Can you work these out from the model? Positions are in its coordinate system, mm. Face numbers are marked on the shaded views. Give positions to 0.01 mm unless a question says otherwise; leave off trailing zeros. Loops run counter-clockwise (first coordinate to the right, second up) from the corner with the lowest first, then second, coordinate; pieces in that order, holes last. Notation, with made-up numbers: (86, -5.75) - (128, -5.75) arc R19 ccw to (128, 30.25) - close; hole circle Ø10 at (-20.75, 38). An arc over 180 degrees is marked (long way). Answer as a JSON object with one key per item and string values.
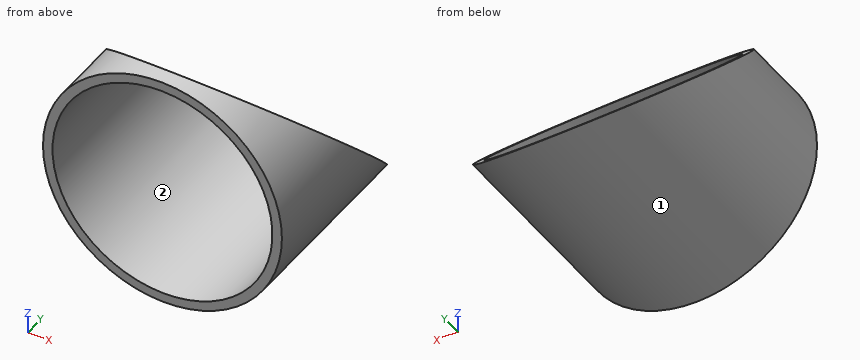
```python
from build123d import *

# Parameters (mm, degrees)
SKETCH2_R               = 20
BOSS_EXTRUDE1_DEPTH     = 0.707106781
SKETCH3_R               = 7.4
SKETCH3_R_2             = 5.9
BOSS_EXTRUDE2_DEPTH     = 1
CUT_EXTRUDE1_DEPTH      = 48.148112734
CUT_EXTRUDE1_DEPTH_BACK = 48.148112734
SKETCH4_W               = 305.220008054
SKETCH4_H               = 126.870977102
SKETCH4_R               = 6.4
BOSS_EXTRUDE3_REACH     = 25.052
SKETCH5_R               = 6.28
SKETCH5_R_2             = 5.78
SKETCH7_R               = 18.282703858
CUT_EXTRUDE3_DEPTH      = 0.707106781
SKETCH8_R               = 12.772794789
CUT_EXTRUDE4_DEPTH      = 2.52


with BuildPart() as part:
    # Sketch2 → Boss-Extrude1 (new body)
    with BuildSketch(Plane(origin=(0, 0, 0), x_dir=(1, 0, 0), z_dir=(0, 0.7071067811865464, 0.7071067811865488))):
        with Locations(Location((0, 20, 0), (0, 0, 270))):
            Circle(SKETCH2_R)
    extrude(amount=-BOSS_EXTRUDE1_DEPTH)

    # Sketch4 → Cut-Extrude1 (cut, two sides: drawn at the far end of the back side and taken through both)
    with BuildSketch(Plane.XZ.offset(3.25).offset(-CUT_EXTRUDE1_DEPTH_BACK)):
        with Locations((6.754756468, -15.87939177)):
            Rectangle(SKETCH4_W, SKETCH4_H)
        with Locations(Location((0, -7.4, 0), (0, 0, 90))):
            Circle(SKETCH4_R, mode=Mode.SUBTRACT)
    extrude(amount=CUT_EXTRUDE1_DEPTH + CUT_EXTRUDE1_DEPTH_BACK, mode=Mode.SUBTRACT)

    # Sketch7 → Cut-Extrude3 (cut)
    with BuildSketch(Plane(origin=(0, 0, 0), x_dir=(1, 0, 0), z_dir=(0, 0.7071067811865465, 0.7071067811865487))):
        with Locations((0, 10.465180362)):
            Circle(SKETCH7_R)
    extrude(amount=-CUT_EXTRUDE3_DEPTH, mode=Mode.SUBTRACT)


with BuildPart() as body_2:
    # Sketch3 → Boss-Extrude2 (new body)
    with BuildSketch(Plane(origin=(0, -3.25, 0), x_dir=(1, 0, 0), z_dir=(0, 1, 0))):
        with Locations(Location((0, 7.4, 0), (0, 0, 270))):
            Circle(SKETCH3_R)
        with Locations(Location((0, 7.4, 0), (0, 0, 270))):
            Circle(SKETCH3_R_2, mode=Mode.SUBTRACT)
    extrude(amount=BOSS_EXTRUDE2_DEPTH)


with BuildPart() as body_3:
    # Boss-Extrude3: up to this plane
    boss_extrude3_end = Plane(origin=(0, 13.642135624, -14.642135624), z_dir=(0, 0.7071067811865464, 0.7071067811865488))
    # Sketch5 → Boss-Extrude3 (new, up to the surface)
    with BuildSketch(Plane(origin=(0, -2.25, 0), x_dir=(1, 0, 0), z_dir=(0, 1, 0)), mode=Mode.PRIVATE) as boss_extrude3_sk1:
        with Locations(Location((0, 7.4, 0), (0, 0, 270))):
            Circle(SKETCH5_R)
        with Locations(Location((0, 7.4, 0), (0, 0, 270))):
            Circle(SKETCH5_R_2, mode=Mode.SUBTRACT)
    boss_extrude3_tool1 = split(extrude(boss_extrude3_sk1.sketch, amount=BOSS_EXTRUDE3_REACH, mode=Mode.PRIVATE), bisect_by=boss_extrude3_end, keep=Keep.BOTH, mode=Mode.PRIVATE)
    add(boss_extrude3_tool1.solids().sort_by_distance((0, -2.25, -13.502375))[0])


with BuildPart() as cut_extrude4_tool:
    # Sketch8 → Cut-Extrude4 (new body)
    with BuildSketch(Plane.XZ.offset(3.25)):
        with Locations((0, -7.395337102)):
            Circle(SKETCH8_R)
    extrude(amount=-CUT_EXTRUDE4_DEPTH)


with BuildPart() as body_2_1:
    add(body_2.part)

    # Cut-Extrude4: cut by cut_extrude4_tool
    add(cut_extrude4_tool.part, mode=Mode.SUBTRACT)


with BuildPart() as body_3_1:
    add(body_3.part)

    # Cut-Extrude4: cut by cut_extrude4_tool
    add(cut_extrude4_tool.part, mode=Mode.SUBTRACT)


solid = body_3_1.part
```
1) I'm going to push flat-ended pins straight in: P1, Ø6, axis at y = 2, z = -9, coming from the +X side; P2, Ø2, axis at x = -2, y = 6.5, coming from the -Z side; P3, Ø5, axis at x = -2, z = -12, coming from the +Y side. Where does each tip first touch, or does it pass through?
Check sheet entries:
{"P1": "x = 6.28", "P2": "z = -13.6", "P3": "y = 12.68"}
2) Imagine slicing it at A-A on x = 0. Write out the boundary of the cut face in (y, z), and give its area (3 significant figures).
Check sheet entries:
{"outline": "(-0.73, -13.68) - (12.68, -13.68) - (12.18, -13.18) - (-0.73, -13.18) - close; (-0.73, -1.62) - (0.62, -1.62) - (0.12, -1.12) - (-0.73, -1.12) - close", "area": "7.13 mm2"}
3) Imagine slicing it at D-D on y = 4.75. Write out the boundary of the cut face in (x, z).
Check sheet entries:
{"outline": "(-6.06, -5.75) arc R6.28 ccw (long way) to (6.06, -5.75) - (5.54, -5.75) arc R5.78 cw (long way) to (-5.54, -5.75) - close"}
4) Imagine slicing it at B-B on z = -7.4. Write out the boundary of the cut face in (x, y).
Check sheet entries:
{"outline": "(-6.28, -0.73) - (-5.78, -0.73) - (-5.78, 6.4) - (-6.28, 6.4) - close; (5.78, -0.73) - (6.28, -0.73) - (6.28, 6.4) - (5.78, 6.4) - close"}
5) I need wall thicknesses on L1, parallel to X at y = 4.25, z = -7.4; L2, parallel to X at y = 6.5, z = -11; L3, parallel to Z at x = 0, y = 7. Which ranges of each line are inside material? Lowest first, please.
Check sheet entries:
{"L1": "-6.28 to -5.78, 5.78 to 6.28", "L2": "-5.15 to -4.52, 4.52 to 5.15", "L3": "-13.68 to -13.18"}
6) Imagine slicing it at C-C on y = 2. Write out the boundary of the cut face in (x, z), and give its area (3 significant figures).
Check sheet entries:
{"outline": "(-4.48, -3) arc R6.28 ccw (long way) to (4.48, -3) - (3.75, -3) arc R5.78 cw (long way) to (-3.75, -3) - close", "area": "14.4 mm2"}
7) If we mould it in two halves opening along X, with no side actions, what happens to the marked faces 1 and 2? For each: released by +X, released by -X, zero draft, split by the parting line, or undercut.
Check sheet entries:
{"face 1": "split by the parting line", "face 2": "undercut"}
